from build123d import *

# Parameters (mm, degrees)
F0_W     = 50
F0_H     = 40
F1_DEPTH = 40
F2_W     = 10
F2_H     = 20
F3_DEPTH = 50.001
F4_W     = 30
F4_H     = 10
F5_DEPTH = 20.001
F6_W     = 10
F6_H     = 20
F7_DEPTH = 20
F8_W     = 10
F8_H     = 20
F9_DEPTH = 30.001


with BuildPart() as f1:
    # F0 (on Front) → F1 (new body)
    with BuildSketch(Plane.XZ):
        with Locations((25, 20)):
            Rectangle(F0_W, F0_H)
    extrude(amount=F1_DEPTH)

    # F2 (on face) → F3 (cut, through all)
    with BuildSketch(Plane(origin=(0, 0, 0), x_dir=(0, -1, 0), z_dir=(-1, 0, 0))):
        with Locations((5, 30)):
            Rectangle(F2_W, F2_H)
        with Locations((35, 30)):
            Rectangle(F2_W, F2_H)
    extrude(amount=-F3_DEPTH, mode=Mode.SUBTRACT)

    # F4 (on face) → F5 (cut, through all)
    with BuildSketch(Plane.XY.offset(20)):
        with Locations((15, -5)):
            Rectangle(F4_W, F4_H)
        with Locations((15, -35)):
            Rectangle(F4_W, F4_H)
    extrude(amount=-F5_DEPTH, mode=Mode.SUBTRACT)

    # F6 (on face) → F7 (cut, through all)
    with BuildSketch(Plane.XY.offset(40)):
        with Locations((45, -20)):
            Rectangle(F6_W, F6_H)
    extrude(amount=-F7_DEPTH, mode=Mode.SUBTRACT)

    # F8 (on face) → F9 (cut, through all)
    with BuildSketch(Plane.XZ.offset(30)):
        with Locations((5, 30)):
            Rectangle(F8_W, F8_H)
    extrude(amount=-F9_DEPTH, mode=Mode.SUBTRACT)


solid = f1.part
Geometry check sheet. Reference: the model listing, model coordinates, mm. A direction names the side the tool comes from. Round coordinates to 2 decimals unless told otherwise and drop trailing zeros. Loops run counter-clockwise (first coordinate to the right, second up) from the corner with the lowest first, then second, coordinate; pieces in that order, holes last. Notation, with made-up numbers: (37, -31) -> (59, -31) arc R20 cw to (59, 3) -> close; hole circle Ø3 at (31.5, 23). An arc over 180 degrees is marked (long way). Answer as a JSON object with one key per item and string values. Group by question number.
Item 1: Set-up check for faces 1 (the face through (30, -5, 10)), 2 (the face through (30, -35, 10)), 3 (the face through (40, -40, 10)), 4 (the face through (10, -20, 30)), 5 (the face through (40, -20, 30)): record each of +Z, -Z, +X, -X, +Y, -Y from which the full face is reachable in a straight line by a thin tool's end or side.
Item 2: Cross-section at A-A, the plane y = -26. Record the cut outline in (x, z), plus the area to 3 significant figures.
Item 3: Cross-section at C-C, the plane x = 7. Record the cut outline in (y, z), plus the area to 3 significant figures.
Item 4: Depth check by flat-ended pin: pin 1 Ø5 at (y, z) = (-4.5, 9) entering from -X; pin 2 Ø2 at (y, z) = (-21, 32.5) entering from -X; pin 3 Ø1.5 at (x, y) = (33.5, -6.5) entering from +Z. Enter the tip coordinate at first touch or a pass-through.
Item 5: Cross-section at D-D, the plane z = 30. Record the cut outline in (x, y).
Item 6: Cross-section at B-B, the plane z = 12. Record the cut outline in (x, y), plus the area to 3 significant figures.
Item 7: Thickness scan on line 1 along Y through (x, z) = (36.5, 36); line 2 along X through (y, z) = (-21, 35); line 3 along Z through (x, y) = (5, -20). Record the ranges inside material, lowest first.
Determined:
{
 "1": {"face 1": "+Z, -Z, -X, +Y", "face 2": "+Z, -Z, -X, -Y", "face 3": "+Z, -Z, +X, -X, -Y", "face 4": "+Z, -X, +Y, -Y", "face 5": "+Z, +X, +Y, -Y"},
 "2": {"outline": "(0, 0) -> (50, 0) -> (50, 20) -> (40, 20) -> (40, 40) -> (10, 40) -> (10, 20) -> (0, 20) -> close", "area": "1,600 mm²"},
 "3": {"outline": "(-30, 0) -> (-10, 0) -> (-10, 20) -> (-30, 20) -> close", "area": "400 mm²"},
 "4": {"pin 1": "stops at x = 30", "pin 2": "stops at x = 10", "pin 3": "stops at z = 20"},
 "5": {"outline": "(10, -30) -> (40, -30) -> (40, -10) -> (10, -10) -> close"},
 "6": {"outline": "(0, -30) -> (30, -30) -> (30, -40) -> (50, -40) -> (50, 0) -> (30, 0) -> (30, -10) -> (0, -10) -> close", "area": "1,400 mm²"},
 "7": {"line 1": "y = -30 to -10", "line 2": "x = 10 to 40", "line 3": "z = 0 to 20"}
}
